Can you work these out from the model? Positions are in its coordinate system, mm. Give positions to 0.01 mm unless a question says otherwise; leave off trailing zeros. Loops run counter-clockwise (first coordinate to the right, second up) from the corner with the lowest first, then second, coordinate; pieces in that order, holes last. Notation, with made-up numbers: M 39,-6.5 L 69,-6.5 A16 cw 69,8.5 Z; hole C 56,76 d9. An arc over 180 degrees is marked long. Answer as a JSON object with one key per item and string values.
```python
from build123d import *

# Parameters (mm, degrees)
SKETCH_3_R          = 4
EXTRUDE_1_DEPTH     = 3
CUT_EXTRUDE_1_DEPTH = 23.045407821


with BuildPart() as part:
    # ｽｹｯﾁ2 → 回転1 (revolve)
    with BuildSketch(Plane.XY, mode=Mode.PRIVATE) as revolve_1_sk:
        with BuildLine():
            Line((-1.5, 13.5), (-1.5, 0))
            Line((-1.5, 0), (1.5, 0))
            Line((1.5, 0), (1.5, 13.5))
            ThreePointArc((1.5, 13.5), (0, 15), (-1.5, 13.5))
        make_face()
    revolve(revolve_1_sk.sketch.rotate(Axis((0, 0, 0), (1, 0, 0)), 90), axis=Axis((0, 0, 0), (1, 0, 0)))

    # ｽｹｯﾁ3 → ﾎﾞｽ - 押し出し1 (add)
    with BuildSketch(Plane.ZY.offset(1.5)):
        with Locations(Location((0, 0, 0), (0, 0, 180))):
            Circle(SKETCH_3_R)
    extrude(amount=EXTRUDE_1_DEPTH)

    # ｽｹｯﾁ4 → ｶｯﾄ - 押し出し1 (cut, through all)
    with BuildSketch(Plane.ZY.offset(4.5)):
        with BuildLine():
            Line((-1.105949818, 1.05), (1.105949818, 1.05))
            ThreePointArc((1.105949818, 1.05), (0, -1.525), (-1.105949818, 1.05))
        make_face()
    extrude(amount=-CUT_EXTRUDE_1_DEPTH, mode=Mode.SUBTRACT)


solid = part.part
```
1) If we mould it in two halves opening along Y, with no side actions, what happens to faces 1 (the cylindrical face through (-1.542, -1.524, 0.05)), 2 (the flat face through (-2, 1.05, 0)), 3 (the flat face through (-1.5, -3, 3)), 4 (the cylindrical face through (-2.979, 3.905, 0.867))? For each: +Y half, -Y half, draft (parallel to the pull), parting line (faces both ways), or undercut.
Answer list:
{"face 1": "undercut", "face 2": "undercut", "face 3": "draft", "face 4": "parting line"}
2) Suppose I cut it at C-C, the plane x = -2.55. Write out the boundary of the cut face in (y, z) (3 decimals).
Answer list:
{"outline": "C 0,0 d8; hole M 1.05,-1.106 L 1.05,1.106 A1.525 ccw long Z"}
3) Suppose I cut it at B-B, the plane y = 0. Write out the boundary of the cut face in (x, z) (3 decimals), and give its area (3 significant figures).
Answer list:
{"outline": "M -4.5,-4 L -1.5,-4 L -1.5,-13.5 A1.5 ccw 1.5,-13.5 L 1.5,-1.525 L -4.5,-1.525 Z; M -4.5,1.525 L 1.5,1.525 L 1.5,13.5 A1.5 ccw -1.5,13.5 L -1.5,4 L -4.5,4 Z", "area": "93.8 mm^2"}
4) Please list where these lines run through material, in increasing order: line 1 along Y through (x, z) = (-1.8, 0) (3 decimals); line 2 along X through (y, z) = (5.5, -7); line 3 along Y through (x, z) = (-1.05, -4.5). Write a range as from..to.
Answer list:
{"line 1": "-4..-1.525, 1.05..4", "line 2": "-1.5..1.5", "line 3": "-13.86..13.86"}
5) Suppose I cut it at D-D, the plane x = -0.2. Write out the boundary of the cut face in (y, z) (3 decimals).
Answer list:
{"outline": "C 0,0 d29.973; hole M 1.05,-1.106 L 1.05,1.106 A1.525 ccw long Z"}
6) Will this pin go through, and if not, where does the flat tip stop? pin 1 Ø0.7 at (x, z) = (-2.5, -0.5) entering from -Y.
Answer list:
{"pin 1": "y = -4"}
7) Suppose I cut it at A-A, the plane z = 0. Write out the boundary of the cut face in (x, y) (3 decimals).
Answer list:
{"outline": "M -4.5,-4 L -1.5,-4 L -1.5,-13.5 A1.5 ccw 1.5,-13.5 L 1.5,-1.525 L -4.5,-1.525 Z; M -4.5,1.05 L 1.5,1.05 L 1.5,13.5 A1.5 ccw -1.5,13.5 L -1.5,4 L -4.5,4 Z"}
